Answer from the drawing. Dimensions are ordinates in mm from the lowest x, y and z of the part. Round coordinates to 2 decimals unless told otherwise and drop trailing zeros. Write each loop counter-clockwise with the first axis right and the second up, starting at its lowest first coordinate (ties: lowest second). Pieces come first, ordered by that corner, then holes.
1. Flat-ended cylindrical pins translate along their axes: pin 1 Ø1 at (x, z) = (4, 17) entering from +Y (1 decimal); pin 2 Ø1.6 at (x, z) = (2.5, 21) entering from -Y; pin 3 Ø1.5 at (y, z) = (5, 23.5) entering from +X; pin 4 Ø2 at (x, y) = (9.5, 7) entering from +Z. Find the tip coordinate at first contact, or state that the pin passes through.
2. Find section A-A (y = 8.75). Write down the section's boundary in (x, z).
3. Find section C-C (x = 10). Write down the section's boundary in (y, z) (1 decimal).
4. Determine the mould class of the marked faces 1, 2, 3 and 4 for opening direction X: pulls with the +X half, pulls with the -X half, needs draft (parallel to the pull), parting line crosses it, or undercut.
5. Find section B-B (z = 19.5). Write down the section's boundary in (x, y) (1 decimal).
6. Straight lines are drawn through the part: probe 1 along X at (y, z) = (9, 7); probe 2 along X at (y, z) = (8.25, 9.5) (1 decimal); probe 3 along Y at (x, z) = (10.25, 4.5) (1 decimal). For each, find the intervals that lie inside material, in ascending order.
7. Find section D-D (x = 11.5). Write down the section's boundary in (y, z).
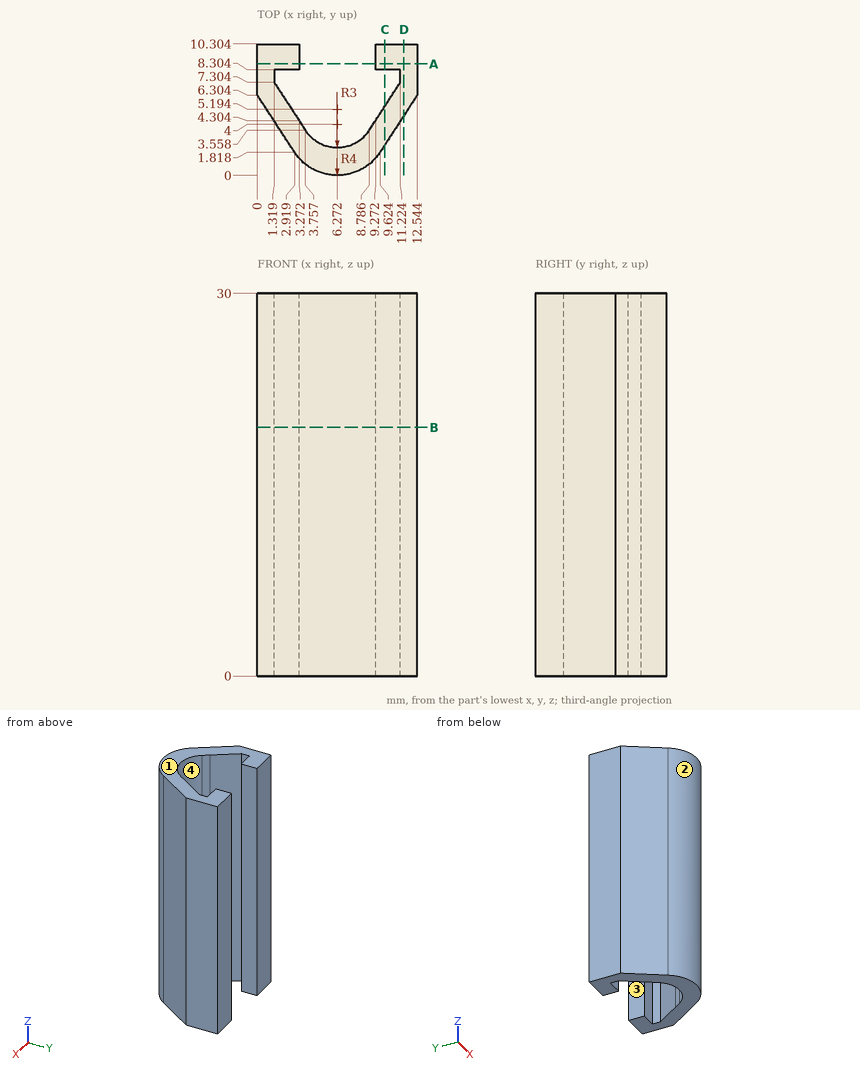
Worked answers:
1. pin 1: stops at y = 4
1. pin 2: stops at y = 1.32
1. pin 3: stops at x = 12.18
1. pin 4: passes through
2. outline: (0, 0) - (3.27, 0) - (3.27, 30) - (0, 30) - close; (9.27, 0) - (12.54, 0) - (12.54, 30) - (9.27, 30) - close
3. outline: (2.4, 0) - (5.4, 0) - (5.4, 30) - (2.4, 30) - close; (8.3, 0) - (10.3, 0) - (10.3, 30) - (8.3, 30) - close
4. face 1: needs draft
4. face 2: parting line crosses it
4. face 3: undercut
4. face 4: undercut
5. outline: (0, 6.3) - (2.9, 1.8) arc R4 ccw to (9.6, 1.8) - (12.5, 6.3) - (12.5, 10.3) - (9.3, 10.3) - (9.3, 8.3) - (11.2, 8.3) - (11.2, 7.3) - (8.8, 3.6) arc R3 cw to (3.8, 3.6) - (1.3, 7.3) - (1.3, 8.3) - (3.3, 8.3) - (3.3, 10.3) - (0, 10.3) - close
6. probe 1: x = 0 to 3.27, 9.27 to 12.54
6. probe 2: x = 0 to 1.3, 11.2 to 12.5
6. probe 3: y = 2.8 to 5.8, 8.3 to 10.3
7. outline: (4.7, 0) - (10.3, 0) - (10.3, 30) - (4.7, 30) - close
